Here's how the part is built. I have some questions about the finished solid (model axes, mm). A direction names the side the tool comes from. Coordinates: 2 decimals unless noted, no trailing zeros. Loops run counter-clockwise (first coordinate to the right, second up) from the corner with the lowest first, then second, coordinate; pieces in that order, holes last. Notation, with made-up numbers: (35, 55.25) -> (41, 55.25) arc R29 ccw to (41, 87.25) -> close; hole circle Ø11 at (81, 26). An arc over 180 degrees is marked (long way). Answer as a JSON object with one key per item and string values. Group by question number.
1) I need wall thicknesses on probe 1 along Z at (x, y) = (139.7, 2); probe 2 along X at (y, z) = (1.75, -10); probe 3 along Z at (x, y) = (88, 1.75). Which ranges of each line are inside material? Lowest first, please. Write a range as [from, to].
2) I want a section at A-A (z = -76.2). Write out the boundary of the cut face in (x, y), then the cut area to 3 significant figures.
3) If we mould it in two halves opening along X, with no side actions, what happens to faces 1 (the cylindrical face through (1.81, 3.22, -112.39)), 2 (the cylindrical face through (59.36, 3.13, -40.44)), 3 (the flat face through (241.3, 3, -56))? For each: +X half, -X half, draft (parallel to the pull), parting line (faces both ways), or undercut.
4) I want a section at D-D (x = 41.5). Write out the boundary of the cut face in (y, z), then the cut area to 3 significant figures.
5) I want a section at B-B (x = 139.7). Write out the boundary of the cut face in (y, z).
6) I want a section at C-C (x = 190.5). Write out the boundary of the cut face in (y, z).
7) Which directions (+Z, -Z, +X, -X, +Y, -Y) give clear straight access to the entire face, cutting with the end or side of a thin tool? Please do faces 4 (the cylindrical face through (190.54, 3.13, -70.96)), 5 (the flat face through (119, 3, 0)).
8) I'm going to push a flat-ended pin straight in: pin 1 (5.5 mm diameter, centred on x = 139.7, z = -104.775, fed in from -Y). Where does the tip first touch, or does it pass through?
```python
from build123d import *

# Parameters (mm, degrees)
SKETCH1_W           = 241.3
SKETCH1_H           = 114.3
SKETCH1_R           = 12.7
SKETCH1_R_2         = 3.175
BOSS_EXTRUDE1_DEPTH = 6.35
FILLET1_R           = 6.35
FILLET2_R           = 1.5875


with BuildPart() as part:
    # Sketch1 → Boss-Extrude1 (new body)
    with BuildSketch(Plane(origin=(0, 0, 0), x_dir=(1, 0, 0), z_dir=(0, 1, 0))):
        with Locations((120.65, 57.15)):
            Rectangle(SKETCH1_W, SKETCH1_H)
        with Locations(Location((38.1, 57.15, 0), (0, 0, 270))):
            Circle(SKETCH1_R, mode=Mode.SUBTRACT)
        with Locations(Location((88.9, 104.775, 0), (0, 0, 270))):
            Circle(SKETCH1_R_2, mode=Mode.SUBTRACT)
        with Locations(Location((139.7, 104.775, 0), (0, 0, 270))):
            Circle(SKETCH1_R_2, mode=Mode.SUBTRACT)
        with Locations(Location((139.7, 9.525, 0), (0, 0, 270))):
            Circle(SKETCH1_R_2, mode=Mode.SUBTRACT)
        with Locations(Location((88.9, 9.525, 0), (0, 0, 270))):
            Circle(SKETCH1_R_2, mode=Mode.SUBTRACT)
        with Locations(Location((18.983968606, 76.2, 0), (0, 0, 270))):
            Circle(SKETCH1_R_2, mode=Mode.SUBTRACT)
        with Locations(Location((18.983968606, 38.1, 0), (0, 0, 270))):
            Circle(SKETCH1_R_2, mode=Mode.SUBTRACT)
        with Locations(Location((57.216031394, 38.1, 0), (0, 0, 270))):
            Circle(SKETCH1_R_2, mode=Mode.SUBTRACT)
        with Locations(Location((57.216031394, 76.2, 0), (0, 0, 270))):
            Circle(SKETCH1_R_2, mode=Mode.SUBTRACT)
        with BuildLine():
            ThreePointArc((188.131704345, 68.331953125), (190.5, 45.72), (192.868295655, 68.331953125))
            ThreePointArc((192.868295655, 68.331953125), (190.5, 70.96125), (188.131704345, 68.331953125))
        make_face(mode=Mode.SUBTRACT)
    extrude(amount=BOSS_EXTRUDE1_DEPTH)

    # Fillet1
    fillet1_edges = [part.edges().sort_by_distance(p)[0] for p in [
        (0, 3.175, -114.3),
        (241.3, 3.175, -114.3),
        (241.3, 3.175, 0),
        (0, 3.175, 0),
    ]]
    fillet(fillet1_edges, radius=FILLET1_R)

    # Fillet2
    fillet2_edges = [part.edges().sort_by_distance(p)[0] for p in [
        (192.868295655, 3.175, -68.331953125),
        (188.131704345, 3.175, -68.331953125),
    ]]
    fillet(fillet2_edges, radius=FILLET2_R)


solid = part.part
```
Determined:
{
 "1": {"probe 1": "[-114.3, -107.95], [-101.6, -12.7], [-6.35, 0]", "probe 2": "[0, 85.76], [92.04, 136.56], [142.84, 241.3]", "probe 3": "[-114.3, -107.82], [-101.73, -12.57], [-6.48, 0]"},
 "2": {"outline": "(0, 0) -> (15.81, 0) -> (15.81, 6.35) -> (0, 6.35) -> close; (22.16, 0) -> (54.04, 0) -> (54.04, 6.35) -> (22.16, 6.35) -> close; (60.39, 0) -> (241.3, 0) -> (241.3, 6.35) -> (60.39, 6.35) -> close", "area": "1,450 mm^2"},
 "3": {"face 1": "-X half", "face 2": "undercut", "face 3": "+X half"},
 "4": {"outline": "(0, -114.3) -> (6.35, -114.3) -> (6.35, -69.39) -> (0, -69.39) -> close; (0, -44.91) -> (6.35, -44.91) -> (6.35, 0) -> (0, 0) -> close", "area": "570 mm^2"},
 "5": {"outline": "(0, -114.3) -> (6.35, -114.3) -> (6.35, -107.95) -> (0, -107.95) -> close; (0, -101.6) -> (6.35, -101.6) -> (6.35, -12.7) -> (0, -12.7) -> close; (0, -6.35) -> (6.35, -6.35) -> (6.35, 0) -> (0, 0) -> close"},
 "6": {"outline": "(0, -114.3) -> (6.35, -114.3) -> (6.35, -70.96) -> (0, -70.96) -> close; (0, -45.72) -> (6.35, -45.72) -> (6.35, 0) -> (0, 0) -> close"},
 "7": {"face 4": "+Y, -Y", "face 5": "+Z, +X, -X, +Y, -Y"},
 "8": {"pin 1": "through"}
}
